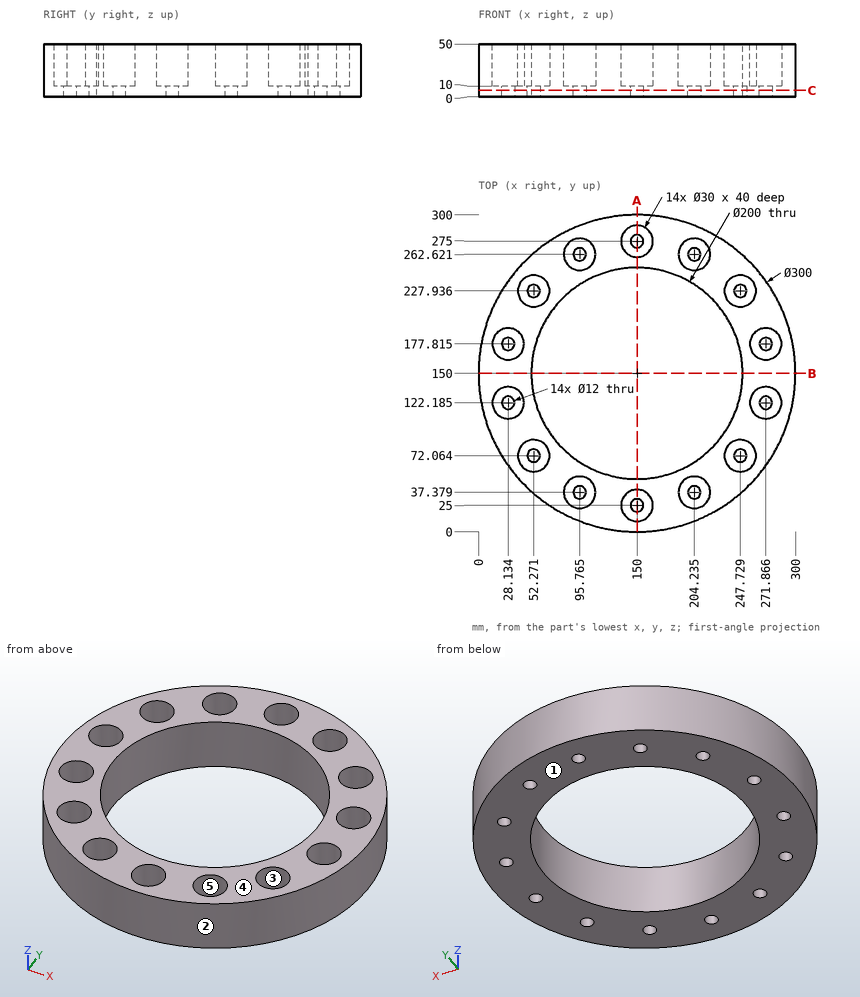
The figure shows three views and two pictorial views of one solid part (mm, origin at its lowest corner). Answer the questions. A direction names the side the tool comes from. Coordinates: 2 decimals unless noted, no trailing zeros. Write each loop counter-clockwise with the first axis right and the second up, starting at its lowest first coordinate (ties: lowest second). Pieces come first, ordered by that corner, then holes.
1. The part is cut by section B-B, the plane y = 150. Write down the section's boundary in (x, z), and give its area (3 significant figures).
Results list:
outline: (0, 0) - (50, 0) - (50, 50) - (0, 50) - close; (250, 0) - (300, 0) - (300, 50) - (250, 50) - close
area: 5,000 mm2
2. For the marked faces 4 and 5, determine the directions among +Z, -Z, +X, -X, +Y, -Y from which every point of the face is accessible in a straight line to the end or side of a thin tool.
Results list:
face 4: +Z, +X, -X, +Y, -Y
face 5: +Z
3. Flat-ended cylindrical pins translate along their axes: pin 1 (24 mm diameter, centred on x = 150, y = 25, fed in from +Z); pin 2 (8 mm diameter, centred on y = 182.5, z = 18, fed in from +X); pin 3 (6 mm diameter, centred on y = 109, z = 19, fed in from +X). Find the tip coordinate at first contact, or state that the pin passes through.
Results list:
pin 1: stops at z = 10
pin 2: stops at x = 297.27
pin 3: stops at x = 295.11
4. The part is cut by section A-A, the plane x = 150. Write down the section's boundary in (y, z), and give its area (3 significant figures).
Results list:
outline: (0, 0) - (19, 0) - (19, 10) - (10, 10) - (10, 50) - (0, 50) - close; (31, 0) - (50, 0) - (50, 50) - (40, 50) - (40, 10) - (31, 10) - close; (250, 0) - (269, 0) - (269, 10) - (260, 10) - (260, 50) - (250, 50) - close; (281, 0) - (300, 0) - (300, 50) - (290, 50) - (290, 10) - (281, 10) - close
area: 2,360 mm2
5. The part is cut by section C-C, the plane z = 6. State how many separate pieces and enclosed holes the cut face has, and give its area (3 significant figures).
Results list:
separate pieces: 1
enclosed holes: 15
area: 37,700 mm2
6. For a pull along Y with two mould halves and no side action, classify the marked faces 1, 2 and 3 as +Y half, -Y half, draft (parallel to the pull), parting line (faces both ways), or undercut.
Results list:
face 1: draft
face 2: parting line
face 3: undercut
7. Consider line 1 along Y through (x, z) = (58, 14) (1 decimal); line 2 along X through (y, z) = (127, 32) (1 decimal); line 3 along Y through (x, z) = (60.5, 15) (1 decimal). Determine where each line is inside the solid, lowest interval first.
Results list:
line 1: y = 31.5 to 58.2, 85.9 to 110.8, 189.2 to 214.1, 241.8 to 268.5
line 2: x = 1.8 to 13.9, 42.3 to 52.7, 247.3 to 257.7, 286.1 to 298.2
line 3: y = 29.6 to 59.5, 84.6 to 105.4, 194.6 to 215.4, 240.5 to 270.4
